from build123d import *

# Parameters (mm, degrees)
BOSS_EXTRUDE1_DEPTH = 7
FILLET1_R           = 2
SKETCH2_R           = 1.5
SKETCH2_R_2         = 1.1
BOSS_EXTRUDE2_DEPTH = 4
SKETCH3_R           = 1.5
SKETCH3_R_2         = 1.1
SKETCH3_W           = 4.5
SKETCH3_H           = 1.5
BOSS_EXTRUDE3_DEPTH = 4


with BuildPart() as part:
    # Sketch1 → Boss-Extrude1 (new body)
    with BuildSketch(Plane(origin=(0, 0, 0), x_dir=(1, 0, 0), z_dir=(0, 1, 0))):
        with BuildLine():
            Line((-10, -9), (10, -9))
            ThreePointArc((10, -9), (11.414213562, -8.414213562), (12, -7))
            Line((12, -7), (12, 7))
            ThreePointArc((12, 7), (11.414213562, 8.414213562), (10, 9))
            Line((10, 9), (-10, 9))
            ThreePointArc((-10, 9), (-11.414213562, 8.414213562), (-12, 7))
            Line((-12, 7), (-12, -7))
            ThreePointArc((-12, -7), (-11.414213562, -8.414213562), (-10, -9))
        make_face()
    extrude(amount=BOSS_EXTRUDE1_DEPTH)

    # Fillet1
    fillet1_edges = [part.edges().sort_by_distance(p)[0] for p in [
        (12, 0, 0),
        (11.414213562, 0, 8.414213562),
        (0, 0, 9),
        (-11.414213562, 0, 8.414213562),
        (11.414213562, 7, 8.414213562),
        (12, 7, 0),
        (11.414213562, 7, -8.414213562),
        (0, 7, -9),
        (-11.414213562, 7, -8.414213562),
        (-12, 7, 0),
        (-11.414213562, 7, 8.414213562),
        (-12, 0, 0),
        (0, 7, 9),
        (-11.414213562, 0, -8.414213562),
        (0, 0, -9),
        (11.414213562, 0, -8.414213562),
    ]]
    fillet(fillet1_edges, radius=FILLET1_R)

    # Sketch2 → Boss-Extrude2 (add)
    with BuildSketch(Plane.ZY.offset(12)):
        with Locations((-7, 3.5)):
            Circle(SKETCH2_R)
        with Locations((-7, 3.5)):
            Circle(SKETCH2_R_2, mode=Mode.SUBTRACT)
        with Locations((0, 3.5)):
            Circle(SKETCH2_R)
        with Locations((0, 3.5)):
            Circle(SKETCH2_R_2, mode=Mode.SUBTRACT)
        with Locations((7, 3.5)):
            Circle(SKETCH2_R)
        with Locations((7, 3.5)):
            Circle(SKETCH2_R_2, mode=Mode.SUBTRACT)
    extrude(amount=BOSS_EXTRUDE2_DEPTH)

    # Sketch3 → Boss-Extrude3 (add)
    with BuildSketch(Plane(origin=(12, 0, 0), x_dir=(0, 0, -1), z_dir=(1, 0, 0))):
        with Locations((-5.167527067, 3.5)):
            Circle(SKETCH3_R)
        with Locations((-5.167527067, 3.5)):
            Circle(SKETCH3_R_2, mode=Mode.SUBTRACT)
        with Locations((-0.767527067, 3.5)):
            Circle(SKETCH3_R)
        with Locations((-0.767527067, 3.5)):
            Circle(SKETCH3_R_2, mode=Mode.SUBTRACT)
        with Locations((5.129819771, 3.5)):
            Rectangle(SKETCH3_W, SKETCH3_H)
    extrude(amount=BOSS_EXTRUDE3_DEPTH)


solid = part.part
Could you check a few things on this model? Use its own coordinates, in mm. A direction names the side the tool comes from. Give positions to 0.01 mm unless a question says otherwise; leave off trailing zeros. Order: outer loops, then holes, each group sorted by start corner. A loop starts at its lowest first (then second) coordinate and runs counter-clockwise, first axis right, second up. Notation, with made-up numbers: (-27, -5) -> (-17, -5) arc R20 cw to (-17, 28) -> close; hole circle Ø4 at (-29.5, 46.25). An arc over 180 degrees is marked (long way). Return JSON: item names as keys, results as strings.
1. Thinking about a two-plate mould opening in Z: for faces 1 (the flat face through (14, 2.75, -5)), 2 (the cylindrical face through (0.14, 6.4, 8.43)), 3 (the flat face through (12, 3, 5)), which applies, pulls with the +Z half, pulls with the -Z half, needs draft (parallel to the pull), parting line crosses it, or undercut?
Answer list:
{"face 1": "needs draft", "face 2": "pulls with the +Z half", "face 3": "undercut"}
2. For pin 1 Ø1.1 at (y, z) = (4, 0) entering from -X; pin 2 Ø1.5 at (y, z) = (3, -1.5) entering from +X; pin 3 Ø0.8 at (x, y) = (14, 3.5) entering from +Z, each with a flat end and sliding along its axis, tell me the tip position at first contact or that it passes through.
Answer list:
{"pin 1": "stops at x = -12", "pin 2": "stops at x = 12", "pin 3": "stops at z = 6.67"}
3. I need wall thicknesses on line 1 (Y direction, x = -15, z = -7); line 2 (X direction, y = 2.5, z = -5.75); line 3 (X direction, y = 4, z = -0.5). Which ranges of each line are inside material? Lowest first, please. Write a range as from..to.
Answer list:
{"line 1": "y = 2..2.4, 4.6..5", "line 2": "x = -12..12", "line 3": "x = -12..16"}
4. Imagine slicing it at B-B on x = -2.5. List the corners of the cut face in (y, z) for me.
Answer list:
{"outline": "(0, -7) arc R2 ccw to (2, -9) -> (5, -9) arc R2 ccw to (7, -7) -> (7, 7) arc R2 ccw to (5, 9) -> (2, 9) arc R2 ccw to (0, 7) -> close"}
5. On a 3-axis mill with a long thin cutter (end or side, diameter ignored), from which of +Z, -Z, +X, -X, +Y, -Y can I reach the whole of each face in a straight line? I mean faces 4 (the flat face through (-12, 3.5, -6.6)), 5 (the flat face through (0, 7, 0)), 6 (the flat face through (12, 3, 3)). Say none if no direction works.
Answer list:
{"face 4": "-X", "face 5": "+Z, -Z, +X, -X, +Y", "face 6": "+X"}
6. Imagine slicing it at C-C on y = 0.5. List the corners of the cut face in (x, z) for me.
Answer list:
{"outline": "(-11.32, -7) arc R1.32 ccw to (-10, -8.32) -> (10, -8.32) arc R1.32 ccw to (11.32, -7) -> (11.32, 7) arc R1.32 ccw to (10, 8.32) -> (-10, 8.32) arc R1.32 ccw to (-11.32, 7) -> close"}
7. Imagine slicing it at A-A on z = -3.5. List the corners of the cut face in (x, y) for me, then the cut area to 3 significant figures.
Answer list:
{"outline": "(-12, 2) arc R2 ccw to (-10, 0) -> (10, 0) arc R2 ccw to (12, 2) -> (12, 2.75) -> (16, 2.75) -> (16, 4.25) -> (12, 4.25) -> (12, 5) arc R2 ccw to (10, 7) -> (-10, 7) arc R2 ccw to (-12, 5) -> close", "area": "171 mm2"}
